Work out the finished part from the listing and answer in its coordinate system (mm). Face numbers are marked on the shaded views. A direction names the side the tool comes from. Give positions to 0.01 mm unless a question says otherwise; leave off trailing zeros. Write each loop counter-clockwise with the first axis right and the second up, starting at its lowest first coordinate (ties: lowest second). Pieces come first, ordered by that corner, then holes.
1) A tool of negligible diameter and unlimited length cuts with its end or side. For the marked faces 1 and 2, from which of +Z, -Z, +X, -X, +Y, -Y can it reach the whole face along a straight path? Write none if from no direction.
2) Find section D-D (x = 69). Determine the outline of the cut face in (y, z), plus the area to 3 significant figures.
3) Straight lines are drawn through the part: probe 1 along X at (y, z) = (1.75, 80); probe 2 along X at (y, z) = (4, 0); probe 3 along Y at (x, z) = (46, 82). For each, find the intervals that lie inside material, in ascending order.
4) Find section A-A (x = 40). Determine the outline of the cut face in (y, z).
5) Find section C-C (z = -14.7). Determine the outline of the cut face in (x, y).
6) Given pin 1 Ø0.6 at (x, y) = (59, 1) entering from -Z; pin 2 Ø2 at (x, y) = (94, 1.5) entering from -Z; pin 3 Ø4 at (x, z) = (94.7, 80) entering from +Y; pin 4 Ø1.7 at (x, z) = (80, 0) entering from +Y (3 decimals), each flat-ended and moving along its own axis, determine where each tip first touches the part or whether it passes through.
7) Find section B-B (y = 4.5). Determine the outline of the cut face in (x, z).
```python
from build123d import *
from OCP.BRepFilletAPI import BRepFilletAPI_MakeChamfer

# Parameters (mm, degrees)
SKIZZE1_W                       = 100
SKIZZE1_H                       = 100
SKIZZE1_R                       = 1.05
AUFSATZ_LINEAR_AUSTRAGEN1_DEPTH = 2
SKIZZE2_R                       = 3
SKIZZE2_R_2                     = 1.05
AUFSATZ_LINEAR_AUSTRAGEN2_DEPTH = 5
VERRUNDUNG1_R                   = 1
FASE1_SIZE                      = 0.8
FASE1_SIZE2                     = 0.953402874
VERRUNDUNG2_R                   = 5
SKIZZE3_W                       = 9.4
SKIZZE3_H                       = 9.4
SKIZZE3_R                       = 1.7
AUFSATZ_LINEAR_AUSTRAGEN3_DEPTH = 2
VERRUNDUNG3_R                   = 3
SKIZZE4_W                       = 9.4
SKIZZE4_H                       = 9.4
SKIZZE4_R                       = 1.7
AUFSATZ_LINEAR_AUSTRAGEN4_DEPTH = 2
VERRUNDUNG4_R                   = 3


with BuildPart() as part:
    # Skizze1 → Aufsatz-Linear austragen1 (new body)
    with BuildSketch(Plane(origin=(0, 0, 0), x_dir=(1, 0, 0), z_dir=(0, 1, 0))):
        with Locations((40, -40)):
            Rectangle(SKIZZE1_W, SKIZZE1_H)
        with Locations(Location((0, 0, 0), (0, 0, 270))):
            Circle(SKIZZE1_R, mode=Mode.SUBTRACT)
        with Locations(Location((0, -80, 0), (0, 0, 270))):
            Circle(SKIZZE1_R, mode=Mode.SUBTRACT)
        with Locations(Location((80, 0, 0), (0, 0, 270))):
            Circle(SKIZZE1_R, mode=Mode.SUBTRACT)
        with Locations(Location((80, -80, 0), (0, 0, 270))):
            Circle(SKIZZE1_R, mode=Mode.SUBTRACT)
    extrude(amount=AUFSATZ_LINEAR_AUSTRAGEN1_DEPTH)

    # Skizze2 → Aufsatz-Linear austragen2 (add)
    # profile 1 of 4: a face of its own
    with BuildSketch(Plane(origin=(0, 2, 0), x_dir=(1, 0, 0), z_dir=(0, 1, 0))):
        with Locations(Location((0, 0, 0), (0, 0, 270))):
            Circle(SKIZZE2_R)
        with Locations(Location((0, 0, 0), (0, 0, 270))):
            Circle(SKIZZE2_R_2, mode=Mode.SUBTRACT)
    # profile 2 of 4: a face of its own
    with BuildSketch(Plane(origin=(0, 2, 0), x_dir=(1, 0, 0), z_dir=(0, 1, 0))):
        with Locations(Location((80, 0, 0), (0, 0, 270))):
            Circle(SKIZZE2_R)
        with Locations(Location((80, 0, 0), (0, 0, 270))):
            Circle(SKIZZE2_R_2, mode=Mode.SUBTRACT)
    # profile 3 of 4: a face of its own
    with BuildSketch(Plane(origin=(0, 2, 0), x_dir=(1, 0, 0), z_dir=(0, 1, 0))):
        with Locations(Location((0, -80, 0), (0, 0, 270))):
            Circle(SKIZZE2_R)
        with Locations(Location((0, -80, 0), (0, 0, 270))):
            Circle(SKIZZE2_R_2, mode=Mode.SUBTRACT)
    # profile 4 of 4: a face of its own
    with BuildSketch(Plane(origin=(0, 2, 0), x_dir=(1, 0, 0), z_dir=(0, 1, 0))):
        with Locations(Location((80, -80, 0), (0, 0, 270))):
            Circle(SKIZZE2_R)
        with Locations(Location((80, -80, 0), (0, 0, 270))):
            Circle(SKIZZE2_R_2, mode=Mode.SUBTRACT)
    extrude(amount=AUFSATZ_LINEAR_AUSTRAGEN2_DEPTH)

    # Verrundung1
    verrundung1_edges = [part.edges().sort_by_distance(p)[0] for p in [
        (0, 2, -3),
        (80, 2, -3),
        (0, 2, 77),
        (80, 2, 77),
    ]]
    fillet(verrundung1_edges, radius=VERRUNDUNG1_R)

    # Fase1: one chamfer whose edges measure the first distance from different faces: ONE call of the kernel's chamfer builder (chamfer() names one face for all edges)
    fase1_edges_1 = [part.edges().sort_by_distance(p)[0] for p in [
        (80, 0, 78.95),
    ]]
    fase1_side_1 = [part.faces().sort_by_distance(p)[0] for p in [
        (80, 3.5, 78.95),
    ]]
    fase1_edges_2 = [part.edges().sort_by_distance(p)[0] for p in [
        (0, 7, -1.05),
    ]]
    fase1_side_2 = [part.faces().sort_by_distance(p)[0] for p in [
        (0, 7, -2.915147186),
    ]]
    fase1_edges_3 = [part.edges().sort_by_distance(p)[0] for p in [
        (80, 7, -1.05),
    ]]
    fase1_side_3 = [part.faces().sort_by_distance(p)[0] for p in [
        (80, 7, -2.915147186),
    ]]
    fase1_edges_4 = [part.edges().sort_by_distance(p)[0] for p in [
        (0, 7, 78.95),
    ]]
    fase1_side_4 = [part.faces().sort_by_distance(p)[0] for p in [
        (0, 7, 77.084852814),
    ]]
    fase1_edges_5 = [part.edges().sort_by_distance(p)[0] for p in [
        (80, 7, 78.95),
    ]]
    fase1_side_5 = [part.faces().sort_by_distance(p)[0] for p in [
        (80, 7, 77.084852814),
    ]]
    fase1 = BRepFilletAPI_MakeChamfer(part.part.solid().wrapped)
    for e in fase1_edges_1:
        fase1.Add(FASE1_SIZE, FASE1_SIZE2, e.wrapped, fase1_side_1[0].wrapped)  # the first distance lies on this face
    for e in fase1_edges_2:
        fase1.Add(FASE1_SIZE, FASE1_SIZE2, e.wrapped, fase1_side_2[0].wrapped)  # the first distance lies on this face
    for e in fase1_edges_3:
        fase1.Add(FASE1_SIZE, FASE1_SIZE2, e.wrapped, fase1_side_3[0].wrapped)  # the first distance lies on this face
    for e in fase1_edges_4:
        fase1.Add(FASE1_SIZE, FASE1_SIZE2, e.wrapped, fase1_side_4[0].wrapped)  # the first distance lies on this face
    for e in fase1_edges_5:
        fase1.Add(FASE1_SIZE, FASE1_SIZE2, e.wrapped, fase1_side_5[0].wrapped)  # the first distance lies on this face
    add(Compound.cast(fase1.Shape()), mode=Mode.REPLACE)

    # Verrundung2
    verrundung2_edges = [part.edges().sort_by_distance(p)[0] for p in [
        (-10, 1, -10),
        (90, 1, -10),
        (90, 1, 90),
        (-10, 1, 90),
    ]]
    fillet(verrundung2_edges, radius=VERRUNDUNG2_R)

    # Skizze3 → Aufsatz-Linear austragen3 (add)
    # profile 1 of 2: a face of its own
    with BuildSketch(Plane(origin=(0, 2, 0), x_dir=(1, 0, 0), z_dir=(0, 1, 0))):
        with Locations((-14.7, -40)):
            Rectangle(SKIZZE3_W, SKIZZE3_H)
        with Locations(Location((-14.7, -40, 0), (0, 0, 270))):
            Circle(SKIZZE3_R, mode=Mode.SUBTRACT)
    # profile 2 of 2: a face of its own
    with BuildSketch(Plane(origin=(0, 2, 0), x_dir=(1, 0, 0), z_dir=(0, 1, 0))):
        with Locations((94.7, -80)):
            Rectangle(SKIZZE3_W, SKIZZE3_H)
        with Locations(Location((94.7, -80, 0), (0, 0, 270))):
            Circle(SKIZZE3_R, mode=Mode.SUBTRACT)
    extrude(amount=-AUFSATZ_LINEAR_AUSTRAGEN3_DEPTH)

    # Verrundung3
    verrundung3_edges = [part.edges().sort_by_distance(p)[0] for p in [
        (90, 1, 84.7),
        (99.4, 1, 84.7),
        (99.4, 1, 75.3),
        (90, 1, 75.3),
        (-10, 1, 35.3),
        (-10, 1, 44.7),
        (-19.4, 1, 44.7),
        (-19.4, 1, 35.3),
    ]]
    fillet(verrundung3_edges, radius=VERRUNDUNG3_R)

    # Skizze4 → Aufsatz-Linear austragen4 (add)
    with BuildSketch(Plane(origin=(0, 2, 0), x_dir=(1, 0, 0), z_dir=(0, 1, 0))):
        with Locations((40, 14.7)):
            Rectangle(SKIZZE4_W, SKIZZE4_H)
        with Locations(Location((40, 14.7, 0), (0, 0, 270))):
            Circle(SKIZZE4_R, mode=Mode.SUBTRACT)
    extrude(amount=-AUFSATZ_LINEAR_AUSTRAGEN4_DEPTH)

    # Verrundung4
    verrundung4_edges = [part.edges().sort_by_distance(p)[0] for p in [
        (44.7, 1, -10),
        (44.7, 1, -19.4),
        (35.3, 1, -19.4),
        (35.3, 1, -10),
    ]]
    fillet(verrundung4_edges, radius=VERRUNDUNG4_R)


solid = part.part
```
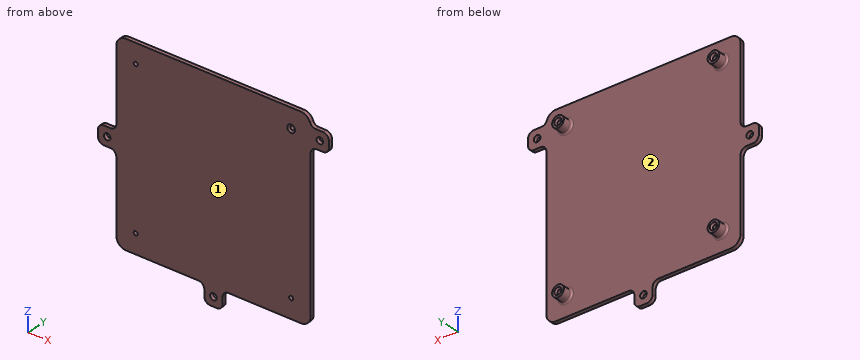
Results:
1. face 1: +Z, -Z, +X, -X, -Y
1. face 2: +Y
2. outline: (0, -10) - (2, -10) - (2, 90) - (0, 90) - close
2. area: 200 mm2
3. probe 1: x = -10 to -1.05, 1.05 to 78.95, 81.05 to 93, 96.4 to 99.4
3. probe 2: x = -3 to -1.05, 1.05 to 3, 77 to 78.95, 81.05 to 83
3. probe 3: y = 0 to 2
4. outline: (0, -19.4) - (2, -19.4) - (2, -16.4) - (0, -16.4) - close; (0, -13) - (2, -13) - (2, 90) - (0, 90) - close
5. outline: (35.3, 0) - (38.3, 0) - (38.3, 2) - (35.3, 2) - close; (41.7, 0) - (44.7, 0) - (44.7, 2) - (41.7, 2) - close
6. pin 1: stops at z = -10
6. pin 2: stops at z = 75.3
6. pin 3: stops at y = 2
6. pin 4: passes through
7. outline: circle Ø6 at (0, 0); circle Ø6 at (0, 80); circle Ø6 at (80, 0); circle Ø6 at (80, 80); hole circle Ø2.1 at (0, 0); hole circle Ø2.1 at (0, 80); hole circle Ø2.1 at (80, 0); hole circle Ø2.1 at (80, 80)
